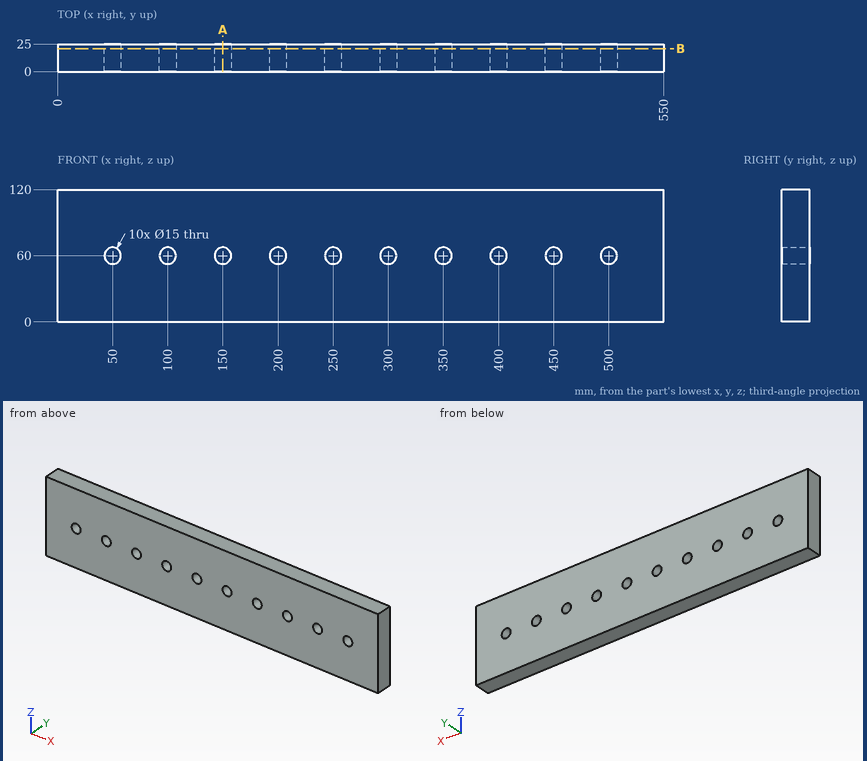
Print and shaded views of the part. All mm, measured from the part's lowest x, y and z. Give positions to 0.01 mm unless a question says otherwise; leave off trailing zeros. Order: outer loops, then holes, each group sorted by start corner. A loop starts at its lowest first (then second) coordinate and runs counter-clockwise, first axis right, second up. Notation, with made-up numbers: (60.5, -4.5) - (69.5, -4.5) arc R23 cw to (69.5, 5.5) - close; hole circle Ø4 at (84, -38). An arc over 180 degrees is marked (long way). Use a Markdown table: item, result.
1) Saw through at B-B on y = 20.75. Count the separate pieces of the cut face and the enclosed holes in it, plus the area to 3 significant figures.
Checked values:
| item | result |
|---|---|
| separate pieces | 1 |
| enclosed holes | 10 |
| area | 64,200 mm² |
2) Flat gauge pin, fed straight in: P1, Ø5, axis at y = 17.5, z = 62, coming from the -X side. Where does the tip first touch, or does it go through?
Checked values:
| item | result |
|---|---|
| P1 | x = 0 |
3) Saw through at A-A on x = 150. List the corners of the cut face in (y, z), plus the area to 4 significant figures.
Checked values:
| item | result |
|---|---|
| outline | (0, 0) - (25, 0) - (25, 52.5) - (0, 52.5) - close; (0, 67.5) - (25, 67.5) - (25, 120) - (0, 120) - close |
| area | 2,625 mm² |
4) Probe L1, parallel to Z at x = 150, y = 13. List the from-to ranges inside material, lowest first. Write a range as from..to.
Checked values:
| item | result |
|---|---|
| L1 | 0..52.5, 67.5..120 |
